Read the model definition and answer for the solid it produces. Units are mm, in the model's axes. A direction names the side the tool comes from. Give positions to 0.01 mm unless a question says otherwise; leave off trailing zeros. Write each loop counter-clockwise with the first axis right and the second up, starting at its lowest first coordinate (ties: lowest second). Pieces come first, ordered by that corner, then holes. Notation, with made-up numbers: M 31,65 L 81,65 A23 ccw 81,93 Z; hole C 77,11 d1. An arc over 180 degrees is marked long. Use a Markdown table: item, result. Add a question column.
Item 1: A cutting plane is placed at C-C on y = 18. Determine the outline of the cut face in (x, z), then the cut area to 3 significant figures.
Item 2: Given P1, Ø1, axis at y = -3.5, z = 2.5, coming from the +X side; P2, Ø1.5, axis at x = -2, z = 4.5, coming from the -Y side; P3, Ø3, axis at y = -9, z = 3.5, coming from the +X side, each flat-ended and moving along its own axis, determine where each tip first touches the part or whether it passes through.
Item 3: A cutting plane is placed at A-A on y = 0. Determine the outline of the cut face in (x, z), then the cut area to 3 significant figures.
Item 4: A cutting plane is placed at D-D on z = 5.5. Determine the outline of the cut face in (x, y), then the cut area to 3 significant figures.
Item 5: For faces 1 (the cylindrical face through (-13.137, 0.578, 4.735)), 2 (the cylindrical face through (-25.5, 0.2, 3.5)), determine the directions among +Z, -Z, +X, -X, +Y, -Y from which every point of the face is accessible in a straight line to the end or side of a thin tool.
Item 6: Consider probe 1 along X at (y, z) = (23, 5.75); probe 2 along X at (y, z) = (22, 2.5); probe 3 along X at (y, z) = (10.5, 3.75). Determine where each line is inside the solid, lowest interval first. Write a range as [from, to].
Item 7: The mould has two halves that part along Y. Classify faces 3 (the cylindrical face through (-22.5, -13.3, 3.5)), 4 (the cylindrical face through (-14.93, -21.53, 3.55)), 5 (the cylindrical face through (-14.872, 21.523, 3.55)): pulls with the +Y half, pulls with the -Y half, needs draft (parallel to the pull), parting line crosses it, or undercut.
from build123d import *

# Parameters (mm, degrees)
SKETCH_1_R          = 9.65
SKETCH_1_R_2        = 2.3
EXTRUDE_1_DEPTH     = 7.2
SKETCH_3_R          = 13.15
CUT_EXTRUDE_2_DEPTH = 5


with BuildPart() as part:
    # Эскиз1 → Бобышка-Вытянуть1 (new body)
    with BuildSketch(Plane.XY):
        with BuildLine():
            ThreePointArc((16.636311976, -22.349119084), (23.768995303, -22.164946702), (23.455168213, -15.036791017))
            ThreePointArc((23.455168213, -15.036791017), (22.512808868, -13.361377812), (22.780834847, -11.457903983))
            ThreePointArc((22.780834847, -11.457903983), (25.5, 0), (22.780834847, 11.457903983))
            ThreePointArc((22.780834847, 11.457903983), (22.512808868, 13.361377812), (23.455168213, 15.036791017))
            ThreePointArc((23.455168213, 15.036791017), (23.768995303, 22.164946702), (16.636311976, 22.349119084))
            ThreePointArc((16.636311976, 22.349119084), (14.899244328, 21.525926197), (13.019103812, 21.9260789))
            ThreePointArc((13.019103812, 21.9260789), (0, 25.5), (-13.019103812, 21.9260789))
            ThreePointArc((-13.019103812, 21.9260789), (-14.899244328, 21.525926197), (-16.636311976, 22.349119084))
            ThreePointArc((-16.636311976, 22.349119084), (-23.768995303, 22.164946702), (-23.455168213, 15.036791017))
            ThreePointArc((-23.455168213, 15.036791017), (-22.512808868, 13.361377812), (-22.780834847, 11.457903983))
            ThreePointArc((-22.780834847, 11.457903983), (-25.5, 0), (-22.780834847, -11.457903983))
            ThreePointArc((-22.780834847, -11.457903983), (-22.512808868, -13.361377812), (-23.455168213, -15.036791017))
            ThreePointArc((-23.455168213, -15.036791017), (-23.768995303, -22.164946702), (-16.636311976, -22.349119084))
            ThreePointArc((-16.636311976, -22.349119084), (-14.899244328, -21.525926197), (-13.019103812, -21.9260789))
            ThreePointArc((-13.019103812, -21.9260789), (0, -25.5), (13.019103812, -21.9260789))
            ThreePointArc((13.019103812, -21.9260789), (14.899244328, -21.525926197), (16.636311976, -22.349119084))
        make_face()
        Circle(SKETCH_1_R, mode=Mode.SUBTRACT)
        with Locations((-20.112226795, -18.754954902)):
            Circle(SKETCH_1_R_2, mode=Mode.SUBTRACT)
        with Locations((20.112226795, -18.754954902)):
            Circle(SKETCH_1_R_2, mode=Mode.SUBTRACT)
        with Locations((20.112226795, 18.754954902)):
            Circle(SKETCH_1_R_2, mode=Mode.SUBTRACT)
        with Locations((-20.112226795, 18.754954902)):
            Circle(SKETCH_1_R_2, mode=Mode.SUBTRACT)
    extrude(amount=EXTRUDE_1_DEPTH)

    # Эскиз3 → Вырез-Вытянуть2 (cut)
    with BuildSketch(Plane.XY.offset(7.2)):
        Circle(SKETCH_3_R)
    extrude(amount=-CUT_EXTRUDE_2_DEPTH, mode=Mode.SUBTRACT)


solid = part.part
Filled in:
| question | item | result |
|---|---|---|
| 1 | outline | M -25.05,0 L -22.28,0 L -22.28,7.2 L -25.05,7.2 Z; M -17.94,0 L 17.94,0 L 17.94,7.2 L -17.94,7.2 Z; M 22.28,0 L 25.05,0 L 25.05,7.2 L 22.28,7.2 Z |
| 1 | area | 298 mm² |
| 2 | P1 | x = 25.32 |
| 2 | P2 | y = -25.47 |
| 2 | P3 | x = 24.37 |
| 3 | outline | M -25.5,0 L -9.65,0 L -9.65,2.2 L -13.15,2.2 L -13.15,7.2 L -25.5,7.2 Z; M 9.65,0 L 25.5,0 L 25.5,7.2 L 13.15,7.2 L 13.15,2.2 L 9.65,2.2 Z |
| 3 | area | 193 mm² |
| 4 | outline | M -23.46,-15.04 A5 ccw long -16.64,-22.35 A3 cw -13.02,-21.93 A25.5 ccw 13.02,-21.93 A3 cw 16.64,-22.35 A5 ccw long 23.46,-15.04 A3 cw 22.78,-11.46 A25.5 ccw 22.78,11.46 A3 cw 23.46,15.04 A5 ccw long 16.64,22.35 A3 cw 13.02,21.93 A25.5 ccw -13.02,21.93 A3 cw -16.64,22.35 A5 ccw long -23.46,15.04 A3 cw -22.78,11.46 A25.5 ccw -22.78,-11.46 A3 cw Z; hole C -20.11,-18.75 d4.6; hole C -20.11,18.75 d4.6; hole C 0,0 d26.3; hole C 20.11,-18.75 d4.6; hole C 20.11,18.75 d4.6 |
| 4 | area | 1,680 mm² |
| 5 | face 1 | +Z |
| 5 | face 2 | +Z, -Z, -X |
| 6 | probe 1 | [-22.75, -17.47], [-11.01, 11.01], [17.47, 22.75] |
| 6 | probe 2 | [-23.92, -16.2], [-12.89, 12.89], [16.2, 23.92] |
| 6 | probe 3 | [-23.24, -7.92], [7.92, 23.24] |
| 7 | face 3 | undercut |
| 7 | face 4 | pulls with the -Y half |
| 7 | face 5 | pulls with the +Y half |
